Geometry check sheet. Reference: the model listing, model coordinates, mm. A direction names the side the tool comes from. Coordinates: 2 decimals unless noted, no trailing zeros. Write each loop counter-clockwise with the first axis right and the second up, starting at its lowest first coordinate (ties: lowest second). Pieces come first, ordered by that corner, then holes. Notation, with made-up numbers: M 28,14 L 35,14 A26 ccw 35,51 Z; hole C -19.5,72.25 d3. An arc over 180 degrees is marked long. Write item = value, one per line. Start each with the question number.
```python
from build123d import *

# Parameters (mm, degrees)
ESQUISSE1_W             = 95
ESQUISSE1_H             = 65
BOSS_EXTRU_1_DEPTH      = 4
ESQUISSE2_R             = 1.7
ENL_V_MAT_EXTRU_1_DEPTH = 5
ESQUISSE3_R             = 2
ENL_V_MAT_EXTRU_2_DEPTH = 3


with BuildPart() as part:
    # Esquisse1 → Boss.-Extru.1 (new body)
    with BuildSketch(Plane.XY):
        Rectangle(ESQUISSE1_W, ESQUISSE1_H)
    extrude(amount=BOSS_EXTRU_1_DEPTH)

    # Esquisse2 → Enlèv. mat.-Extru.1 (cut)
    with BuildSketch(Plane(origin=(0, 0, 0), x_dir=(-1, 0, 0), z_dir=(0, 0, -1))):
        with Locations((-41.5, 26.5)):
            Circle(ESQUISSE2_R)
        with Locations(Location((41.5, 26.5, 0), (0, 0, 180))):
            Circle(ESQUISSE2_R)
        with Locations(Location((-41.5, -26.5, 0), (0, 0, 180))):
            Circle(ESQUISSE2_R)
        with Locations((41.5, -26.5)):
            Circle(ESQUISSE2_R)
    extrude(amount=-ENL_V_MAT_EXTRU_1_DEPTH, mode=Mode.SUBTRACT)

    # Esquisse3 → Enlèv. mat.-Extru.2 (cut)
    with BuildSketch(Plane.XY.offset(4)):
        with Locations((18.5, 25.96)):
            Circle(ESQUISSE3_R)
        with Locations((-33.57, 20.88)):
            Circle(ESQUISSE3_R)
        with Locations((-33.57, -7.06)):
            Circle(ESQUISSE3_R)
    extrude(amount=-ENL_V_MAT_EXTRU_2_DEPTH, mode=Mode.SUBTRACT)


solid = part.part
```
Q1. Set-up check for faces 5 (the face through (-34, 21, 1)), 6 (the face through (42.75, 27.65, 1.97)): record each of +Z, -Z, +X, -X, +Y, -Y from which the full face is reachable in a straight line by a thin tool's end or side.
Q2. Cross-section at B-B on x = -33.57. Enter the section's corners in (y, z), and give its area (3 significant figures).
Q3. Scan lines: L1, parallel to Y at x = 41.5, z = 2.7; L2, parallel to Y at x = 18.5, z = 2.4; L3, parallel to X at y = -25, z = 0.9. Record each from-to range of solid material in increasing order.
Q4. Cross-section at C-C on x = 18.5. Enter the section's corners in (y, z), and give its area (3 significant figures).
Q5. Cross-section at A-A on y = -26.5. Enter the section's corners in (x, z), and give its area (3 significant figures).
Q6. Draft check along Y on faces 1 (the face through (-1, -32.5, 2)), 2 (the face through (-40.25, -25.35, 1.97)), 3 (the face through (-1, 0, 4)), 4 (the face through (40.25, -27.65, 1.97)). Enter one of: pulls with the +Y half, pulls with the -Y half, needs draft (parallel to the pull), parting line crosses it, or undercut.
Q7. Gauge pin test, flat ends, axial feed: pin 1 (2 mm diameter, centred on x = 41.5, y = -26.5, fed in from +Z); pin 2 (5 mm diameter, centred on x = 18.5, y = 25.96, fed in from -Z); pin 3 (1.2 mm diameter, centred on x = 19, y = 26.5, fed in from +Z). Record the tip position at first contact, or that the pin passes through.
Values found:
q1.face_5 = +Z
q1.face_6 = +Z, -Z
q2.outline = M -32.5,0 L 32.5,0 L 32.5,4 L 22.88,4 L 22.88,1 L 18.88,1 L 18.88,4 L -5.06,4 L -5.06,1 L -9.06,1 L -9.06,4 L -32.5,4 Z
q2.area = 236 mm²
q3.L1 = -32.5 to -28.2, -24.8 to 24.8, 28.2 to 32.5
q3.L2 = -32.5 to 23.96, 27.96 to 32.5
q3.L3 = -47.5 to -42.3, -40.7 to 40.7, 42.3 to 47.5
q4.outline = M -32.5,0 L 32.5,0 L 32.5,4 L 27.96,4 L 27.96,1 L 23.96,1 L 23.96,4 L -32.5,4 Z
q4.area = 248 mm²
q5.outline = M -47.5,0 L -43.2,0 L -43.2,4 L -47.5,4 Z; M -39.8,0 L 39.8,0 L 39.8,4 L -39.8,4 Z; M 43.2,0 L 47.5,0 L 47.5,4 L 43.2,4 Z
q5.area = 353 mm²
q6.face_1 = pulls with the -Y half
q6.face_2 = undercut
q6.face_3 = needs draft
q6.face_4 = undercut
q7.pin_1 = through
q7.pin_2 = 0
q7.pin_3 = 1
